Design review of the part built by this model. Coordinates are the model's own, in mm. A direction names the side the tool comes from. Coordinates: 2 decimals unless noted, no trailing zeros. Loops run counter-clockwise (first coordinate to the right, second up) from the corner with the lowest first, then second, coordinate; pieces in that order, holes last. Notation, with made-up numbers: (67.5, -28) -> (85.5, -28) arc R13 cw to (85.5, -9) -> close; hole circle Ø5 at (18, -6.75). An arc over 180 degrees is marked (long way). Use a Markdown table: item, result. Add a question column.
Q1. Clearance check with flat-ended pins moving along their axes: pin 1 Ø6 at (x, y) = (0, 0) entering from +Z; pin 2 Ø1.5 at (x, z) = (-4, -3) entering from +Y; pin 3 Ø2 at (x, z) = (-5, -2.5) entering from +Y; pin 4 Ø9 at (x, y) = (0, 0) entering from -Z. State where each tip first meets the part, or that it passes through.
Q2. For faces 4 (the face through (0, 0, -2)), 5 (the face through (-2.59, -1.074, -4.553)), list the 3-axis set-ups (+Z, -Z, +X, -X, +Y, -Y) from which the entire face can be reached by the end or side of a thin tool; tool diameter is ignored.
Q3. For probe 1 along Y at (x, z) = (0, -0.35); probe 2 along Z at (x, y) = (1.5, 7.25); probe 3 along Y at (x, z) = (0, -0.9), list the stretches that pass through material, from the lowest coordinate up.
Q4. Draft analysis for pull direction X (two halves, no side actions). For faces 1 (the face through (-5, 2, 0)), 2 (the face through (1.08, -4.88, 0.25)), 3 (the face through (-0.233, -0.096, -3.893)), state which applies: pulls with the +X half, pulls with the -X half, needs draft (parallel to the pull), parting line crosses it, or undercut.
Q5. Take a section at A-A on z = -3.15. Write out the cut boundary in (x, y).
from build123d import *

# Parameters (mm, degrees)
F0_W    = 1
F0_H    = 0.5
F2_R    = 0.3
F3_SIZE = 0.5
F4_SIZE = 0.2


with BuildPart() as f1:
    # F0 (on Front) → F1 (revolve)
    with BuildSketch(Plane.XZ):
        Polygon((-4, -2), (-4, 0), (-5, 0), (-11, 0), (-2, -5), (0, -3.733945), (0, -2), align=None)
        with Locations((-4.5, 0.25)):
            Rectangle(F0_W, F0_H)
    revolve(axis=Axis((0, 0, -1.866972), (0, 0, -1)))

    # F2
    f2_edges = [f1.edges().sort_by_distance(p)[0] for p in [
        (11, 0, 0),
    ]]
    fillet(f2_edges, radius=F2_R)

    # F3
    f3_edges = [f1.edges().sort_by_distance(p)[0] for p in [
        (2, 0, -5),
    ]]
    chamfer(f3_edges, length=F3_SIZE)

    # F4
    f4_edges = [f1.edges().sort_by_distance(p)[0] for p in [
        (4, 0, 0.5),
    ]]
    chamfer(f4_edges, length=F4_SIZE)


solid = f1.part
Answer list:
| question | item | result |
|---|---|---|
| 1 | pin 1 | z = -2 |
| 1 | pin 2 | y = 5.76 |
| 1 | pin 3 | y = 6.74 |
| 1 | pin 4 | z = -4.76 |
| 2 | face 4 | +Z |
| 2 | face 5 | -Z |
| 3 | probe 1 | -10.14 to -4, 4 to 10.14 |
| 3 | probe 2 | -2 to 0 |
| 3 | probe 3 | -9.38 to -4, 4 to 9.38 |
| 4 | face 1 | needs draft |
| 4 | face 2 | parting line crosses it |
| 4 | face 3 | undercut |
| 5 | outline | circle Ø10.66 at (0, 0) |
